Design review of the part built by this model. Coordinates are the model's own, in mm. A direction names the side the tool comes from. Give positions to 0.01 mm unless a question says otherwise; leave off trailing zeros. Write each loop counter-clockwise with the first axis right and the second up, starting at its lowest first coordinate (ties: lowest second). Pieces come first, ordered by that corner, then holes.
```python
from build123d import *

# Parameters (mm, degrees)
SKETCH1_W           = 20
SKETCH1_H           = 20
BOSS_EXTRUDE1_DEPTH = 3
SKETCH2_W           = 3
SKETCH2_H           = 20
BOSS_EXTRUDE2_DEPTH = 150
SKETCH3_W           = 17
SKETCH3_H           = 3
BOSS_EXTRUDE3_DEPTH = 150
SKETCH4_R           = 1.6
CUT_EXTRUDE1_DEPTH  = 3
SKETCH5_W           = 30
SKETCH5_H           = 17
BOSS_EXTRUDE4_DEPTH = 4
SKETCH6_W           = 30
SKETCH6_H           = 17
BOSS_EXTRUDE5_DEPTH = 4
SKETCH9_R           = 2.05
SKETCH9_R_2         = 2.1
CUT_EXTRUDE4_DEPTH  = 186.434844337
SKETCH10_R          = 4
CUT_EXTRUDE5_DEPTH  = 2.5
CHAMFER3_SIZE       = 3
SKETCH12_W          = 3.1
SKETCH12_H          = 17
CUT_EXTRUDE7_DEPTH  = 3


with BuildPart() as part:
    # Sketch1 → Boss-Extrude1 (new body)
    with BuildSketch(Plane(origin=(0, 0, 0), x_dir=(0, 0, -1), z_dir=(1, 0, 0))):
        with Locations((-98.245468701, -9.501201475)):
            Rectangle(SKETCH1_W, SKETCH1_H)
    extrude(amount=BOSS_EXTRUDE1_DEPTH)

    # Sketch2 → Boss-Extrude2 (add)
    with BuildSketch(Plane.ZY):
        with Locations((106.745468701, -9.501201475)):
            Rectangle(SKETCH2_W, SKETCH2_H)
    extrude(amount=BOSS_EXTRUDE2_DEPTH)

    # Sketch3 → Boss-Extrude3 (add)
    with BuildSketch(Plane.ZY):
        with Locations((96.745468701, -18.001201475)):
            Rectangle(SKETCH3_W, SKETCH3_H)
    extrude(amount=BOSS_EXTRUDE3_DEPTH)

    # Sketch4 → Cut-Extrude1 (cut)
    with BuildSketch(Plane(origin=(3, 0, 0), x_dir=(0, 0, -1), z_dir=(1, 0, 0))):
        with Locations((-101.245468701, -4.501201475)):
            Circle(SKETCH4_R)
        with Locations((-92.245468701, -4.501201475)):
            Circle(SKETCH4_R)
        with Locations((-92.245468701, -12.501201475)):
            Circle(SKETCH4_R)
        with Locations((-101.245468701, -12.501201475)):
            Circle(SKETCH4_R)
    extrude(amount=-CUT_EXTRUDE1_DEPTH, mode=Mode.SUBTRACT)

    # Sketch5 → Boss-Extrude4 (add)
    with BuildSketch(Plane(origin=(0, -16.501201475, 0), x_dir=(1, 0, 0), z_dir=(0, 1, 0))):
        with Locations((-135, -96.745468701)):
            Rectangle(SKETCH5_W, SKETCH5_H)
    extrude(amount=BOSS_EXTRUDE4_DEPTH)

    # Sketch6 → Boss-Extrude5 (add)
    with BuildSketch(Plane(origin=(0, -16.501201475, 0), x_dir=(1, 0, 0), z_dir=(0, 1, 0))):
        with Locations((-65, -96.745468701)):
            Rectangle(SKETCH6_W, SKETCH6_H)
    extrude(amount=BOSS_EXTRUDE5_DEPTH)

    # Sketch9 → Cut-Extrude4 (cut, through all)
    with BuildSketch(Plane(origin=(0, -12.501201475, 0), x_dir=(1, 0, 0), z_dir=(0, 1, 0))):
        with Locations(Location((-58, -96.745468701, 0), (0, 0, 270))):
            Circle(SKETCH9_R)
        with Locations(Location((-72, -96.745468701, 0), (0, 0, 270))):
            Circle(SKETCH9_R_2)
        with Locations(Location((-128, -96.745468701, 0), (0, 0, 270))):
            Circle(SKETCH9_R_2)
        with Locations(Location((-142, -96.745468701, 0), (0, 0, 270))):
            Circle(SKETCH9_R_2)
    extrude(amount=-CUT_EXTRUDE4_DEPTH, mode=Mode.SUBTRACT)

    # Sketch10 → Cut-Extrude5 (cut)
    with BuildSketch(Plane.XZ.offset(19.501201475)):
        with Locations(Location((-142, 96.745468701, 0), (0, 0, 270))):
            Circle(SKETCH10_R)
        with Locations(Location((-128, 96.745468701, 0), (0, 0, 270))):
            Circle(SKETCH10_R)
        with Locations(Location((-72, 96.745468701, 0), (0, 0, 270))):
            Circle(SKETCH10_R)
        with Locations(Location((-58, 96.745468701, 0), (0, 0, 270))):
            Circle(SKETCH10_R)
    extrude(amount=-CUT_EXTRUDE5_DEPTH, mode=Mode.SUBTRACT)

    # Chamfer3
    chamfer3_edges = [part.edges().sort_by_distance(p)[0] for p in [
        (-100, -16.501201475, 105.245468701),
        (-25, -16.501201475, 105.245468701),
    ]]
    chamfer(chamfer3_edges, length=CHAMFER3_SIZE)

    # Sketch12 → Cut-Extrude7 (cut)
    with BuildSketch(Plane(origin=(0, -16.501201475, 0), x_dir=(1, 0, 0), z_dir=(0, 1, 0))):
        with Locations((-118.45, -96.745468701)):
            Rectangle(SKETCH12_W, SKETCH12_H)
        with Locations((-81.55, -96.745468701)):
            Rectangle(SKETCH12_W, SKETCH12_H)
        with Locations((-48.45, -96.745468701)):
            Rectangle(SKETCH12_W, SKETCH12_H)
    extrude(amount=CUT_EXTRUDE7_DEPTH, mode=Mode.SUBTRACT)


solid = part.part
```
(1) Consider section B-B, the plane x = -34.5. Give the boundary of the cut face in (y, z).
Resolved:
outline: (-19.5, 88.25) - (-16.5, 88.25) - (-16.5, 102.25) - (-13.5, 105.25) - (0.5, 105.25) - (0.5, 108.25) - (-19.5, 108.25) - close
(2) Consider section A-A, the plane x = -58. Give the boundary of the cut face in (y, z), then the cut area to 3 significant figures.
Resolved:
outline: (-19.5, 88.25) - (-12.5, 88.25) - (-12.5, 94.7) - (-17, 94.7) - (-17, 92.75) - (-19.5, 92.75) - close; (-19.5, 100.75) - (-17, 100.75) - (-17, 98.8) - (-12.5, 98.8) - (-12.5, 105.25) - (0.5, 105.25) - (0.5, 108.25) - (-19.5, 108.25) - close
area: 141 mm2
(3) Tool access review of faces 1 (the face through (-65, -12.501, 97)), 2 (the face through (-25, -16.501, 95)), 3 (the face through (-130, -17.001, 95)), 4 (the face through (1.521, -12.431, 102.844)): name each direction out of +Z, -Z, +X, -X, +Y, -Y from which nothing blocks a thin tool from reaching the whole face with its end or side.
Resolved:
face 1: -Z, -X, +Y
face 2: -Z, +Y
face 3: -Y
face 4: +X
(4) To check wall thickness, follow L1, parallel to Z at x = -142, y = -14.75; L2, parallel to X at y = -3, z = 91; L3, parallel to Z at x = -10, y = -10. State the ranges of each line that lie inside material, in increasing order.
Resolved:
L1: z = 88.25 to 94.65, 98.85 to 108.25
L2: x = 0 to 3
L3: z = 105.25 to 108.25
(5) Mouldability with a two-part tool opening along Y and no side actions: class faces 5 (the face through (-150, -14, 101)), 6 (the face through (1.521, -4.431, 102.844)), 7 (the face through (-99.763, -15.022, 103.724)) as pulls with the +Y half, pulls with the -Y half, needs draft (parallel to the pull), parting line crosses it, or undercut.
Resolved:
face 5: needs draft
face 6: undercut
face 7: pulls with the +Y half
(6) Clearance check with flat-ended pins moving along their axes: P1, Ø6.5, axis at x = -72, z = 96.75, coming from the +Y side; P2, Ø12, axis at y = -4, z = 94.5, coming from the -X side; P3, Ø5, axis at x = -142, z = 96.75, coming from the -Y side. State where each tip first meets the part, or that it passes through.
Resolved:
P1: stops at y = -12.5
P2: stops at x = 0
P3: stops at y = -17
(7) Consider section C-C, the plane y = -8. Give the boundary of the cut face in (x, z), then the cut area to 3 significant figures.
Resolved:
outline: (-150, 105.25) - (0, 105.25) - (0, 88.25) - (3, 88.25) - (3, 108.25) - (-150, 108.25) - close
area: 510 mm2
(8) Consider section D-D, the plane z = 96. Give the number of separate pieces and of enclosed holes in the cut face, then the cut area to 3 significant figures.
Resolved:
separate pieces: 5
enclosed holes: 0
area: 601 mm2
